from build123d import *

# Parameters (mm, degrees)
F1_DEPTH = 5
F2_R     = 2
F3_DEPTH = 25


with BuildPart() as f1:
    # F0 (on Front) → F1 (new body)
    with BuildSketch(Plane.XZ):
        Polygon((35, -25.5), (35, 25.5), (-35, 25.5), (-35, -25.5), (-16, -25.5), (-16, -28.5), (16, -28.5), (16, -25.5), align=None)
    extrude(amount=F1_DEPTH)

    # F2 (on face) → F3 (cut)
    with BuildSketch(Plane.XZ.offset(5)):
        with Locations((-20, 10.5)):
            Circle(F2_R)
        with Locations((20, 10.5)):
            Circle(F2_R)
    extrude(amount=-F3_DEPTH, mode=Mode.SUBTRACT)


solid = f1.part
The listing builds one solid part. Answer for the finished solid, in the listing's coordinates (mm). A direction names the side the tool comes from. Round coordinates to 2 decimals unless told otherwise and drop trailing zeros. Order: outer loops, then holes, each group sorted by start corner. A loop starts at its lowest first (then second) coordinate and runs counter-clockwise, first axis right, second up. Notation, with made-up numbers: (5, -38) -> (36, -38) arc R19 ccw to (36, -19) -> close; hole circle Ø9 at (45.5, 9). An arc over 180 degrees is marked (long way). Put each result on its own line as item: value.
Q1. This flat-tipped pin is pushed along its axis until it touches: P1, Ø1.5, axis at x = 28, y = -3, coming from the -Z side. Where does it stop, or does it pass through?
Results list:
P1: z = -25.5
Q2. Section A-A, the plane z = 10.5 is taken. Write down the section's boundary in (x, y).
Results list:
outline: (-35, -5) -> (-22, -5) -> (-22, 0) -> (-35, 0) -> close; (-18, -5) -> (18, -5) -> (18, 0) -> (-18, 0) -> close; (22, -5) -> (35, -5) -> (35, 0) -> (22, 0) -> close
Q3. Consider line 1 along Z through (x, y) = (20, -1.8); line 2 along Z through (x, y) = (28, -0.25); line 3 along Z through (x, y) = (-21.5, -2.55). Determine where each line is inside the solid, lowest interval first.
Results list:
line 1: -25.5 to 8.5, 12.5 to 25.5
line 2: -25.5 to 25.5
line 3: -25.5 to 9.18, 11.82 to 25.5
Q4. Section C-C, the plane x = 20 is taken. Write down the section's boundary in (y, z), and give its area (3 significant figures).
Results list:
outline: (-5, -25.5) -> (0, -25.5) -> (0, 8.5) -> (-5, 8.5) -> close; (-5, 12.5) -> (0, 12.5) -> (0, 25.5) -> (-5, 25.5) -> close
area: 235 mm^2
Q5. Determine the mould class of faces 4 (the flat face through (16, -2, -27)), 5 (the cylindrical face through (19.74, -2.535, 12.483)), 6 (the flat face through (0, -5, -1)) for opening direction X: pulls with the +X half, pulls with the -X half, needs draft (parallel to the pull), parting line crosses it, or undercut.
Results list:
face 4: pulls with the +X half
face 5: undercut
face 6: needs draft
Q6. Which of the six approach directions +Z, -Z, +X, -X, +Y, -Y give full straight-line access (tool end or side, diameter ignored) to faces 1 (the flat face through (35, -2, 0)), 2 (the flat face through (-16, -2, -27)), 3 (the flat face through (25, -2, -25.5))?
Results list:
face 1: +Z, -Z, +X, +Y, -Y
face 2: -Z, -X, +Y, -Y
face 3: -Z, +X, +Y, -Y
Q7. Section B-B, the plane y = -0.8 is taken. Write down the section's boundary in (x, z), and give its area (3 significant figures).
Results list:
outline: (-35, -25.5) -> (-16, -25.5) -> (-16, -28.5) -> (16, -28.5) -> (16, -25.5) -> (35, -25.5) -> (35, 25.5) -> (-35, 25.5) -> close; hole circle Ø4 at (-20, 10.5); hole circle Ø4 at (20, 10.5)
area: 3,640 mm^2
